Source: CAD feature listing. Evaluate the final solid. Frame: model axes, mm. Give positions to 0.01 mm unless a question says otherwise; leave off trailing zeros. Order: outer loops, then holes, each group sorted by start corner. A loop starts at its lowest first (then second) coordinate and runs counter-clockwise, first axis right, second up. Notation, with made-up numbers: M -15.75,49.5 L 16.25,49.5 A31 cw 16.25,79.5 Z; hole C 54,72 d3. An arc over 180 degrees is marked long. Answer as a JSON object with one key per item and string values. Group by question number.
1. Pull-direction query (X, two-part tool) for faces 1 (the flat face through (8.9, -39.3, 81)), 2 (the cylindrical face through (-8.67, -39.05, 40.44)), 3 (the cylindrical face through (-9, -40, 40)); classes: +X half, -X half, draft (parallel to the pull), parting line (faces both ways), or undercut.
2. Section query C-C (z = 56.5). Output: boundary loops of the cut face in (x, y), plus the area to 3 significant figures.
3. Pin query (flat end, axial travel): P1, Ø12, axis at x = 18, y = -22, coming from the +Z side; P2, Ø2, axis at x = 18, z = 39, coming from the +Y side; P3, Ø1.5, axis at x = -30, z = 25.5, coming from the +Y side; P4, Ø10, axis at y = -19, z = 28, coming from the +X side. Return the tip coordinate at first contact, or that it passes through.
4. Material intervals for L1, parallel to Y at x = 0, z = 22; L2, parallel to X at y = 32.5, z = 70 (3 decimals); L3, parallel to Y at x = -35, z = 44, sorted ascending. Write a range as [from, to].
5. Section query B-B (y = 20). Output: boundary loops of the cut face in (x, z).
6. Section query A-A (x = 0). Output: boundary loops of the cut face in (y, z), plus the area to 3 significant figures.
from build123d import *

# Parameters (mm, degrees)
CYLINDER016_R     = 40
CYLINDER016_DEPTH = 80
CYLINDER017_R     = 41
CYLINDER017_DEPTH = 80


with BuildPart() as cylinder016:
    # Cylinder016 → Cylinder016 (new body)
    with BuildSketch(Plane.XY.offset(1)):
        Circle(CYLINDER016_R)
    extrude(amount=CYLINDER016_DEPTH)


with BuildPart() as cut004:
    # Cylinder017 → Cylinder017 (new body)
    with BuildSketch(Plane.XY.offset(1)):
        Circle(CYLINDER017_R)
    extrude(amount=CYLINDER017_DEPTH)

    # Cut004: cut Cylinder016
    add(cylinder016.part, mode=Mode.SUBTRACT)


solid = cut004.part
Answer sheet:
{
 "1": {"face 1": "draft", "face 2": "undercut", "face 3": "parting line"},
 "2": {"outline": "C 0,0 d82; hole C 0,0 d80", "area": "254 mm^2"},
 "3": {"P1": "through", "P2": "y = 37.31", "P3": "y = 28.73", "P4": "x = 38.54"},
 "4": {"L1": "[-41, -40], [40, 41]", "L2": "[-24.995, -23.318], [23.318, 24.995]", "L3": "[-21.35, -19.36], [19.36, 21.35]"},
 "5": {"outline": "M -35.79,1 L -34.64,1 L -34.64,81 L -35.79,81 Z; M 34.64,1 L 35.79,1 L 35.79,81 L 34.64,81 Z"},
 "6": {"outline": "M -41,1 L -40,1 L -40,81 L -41,81 Z; M 40,1 L 41,1 L 41,81 L 40,81 Z", "area": "160 mm^2"}
}
